Check sheet for the drawn part. Datum: minimum x, y, z corner. Units: mm. Coordinates: 2 decimals unless noted, no trailing zeros. Loops run counter-clockwise (first coordinate to the right, second up) from the corner with the lowest first, then second, coordinate; pieces in that order, holes last. Notation, with made-up numbers: (38.25, 60.25) - (64.25, 60.25) arc R9 cw to (64.25, 74.25) - close; hole circle Ø5 at (-19, 83.5). An arc over 180 degrees is marked (long way). Answer as CSV lines item,"result". Start each with the question number.
1. Gauge pin test, flat end, axial feed: P1, Ø1.8, axis at x = 2.5, y = 2.5, coming from the +Z side. Record the tip position at first contact, or that the pin passes through.
2. Cross-section at A-A (x = 2.5). Enter the section's corners in (y, z), plus the area to 3 significant figures.
3. Cross-section at B-B (z = 0.6). Enter the section's corners in (x, y), plus the area to 3 significant figures.
4. Cross-section at C-C (x = 3.75). Enter the section's corners in (y, z), plus the area to 3 significant figures.
5. Material ranges on line 1 (Y direction, x = 2.5, z = 1.4); line 2 (Y direction, x = 1.35, z = 1.85); line 3 (X direction, y = 3.5, z = 0.65), recorded low to high. Write a range as [from, to].
6. Release check for a two-part mould opening along Y. For the marked faces 1, 2 and 3 record: pulls with the +Y half, pulls with the -Y half, needs draft (parallel to the pull), parting line crosses it, or undercut.
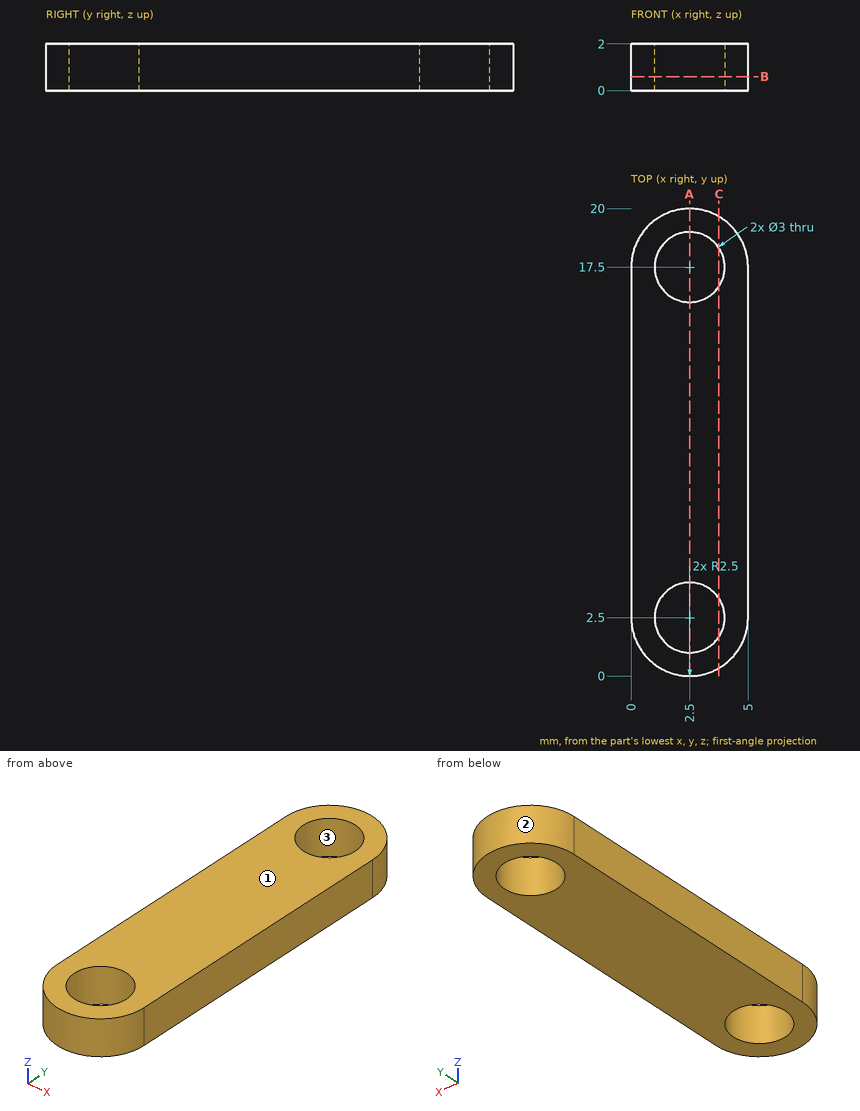
Values follow:
1,P1,"passes through"
2,outline,"(0, 0) - (1, 0) - (1, 2) - (0, 2) - close; (4, 0) - (16, 0) - (16, 2) - (4, 2) - close; (19, 0) - (20, 0) - (20, 2) - (19, 2) - close"
2,area,"28.0 mm²"
3,outline,"(0, 2.5) arc R2.5 ccw to (5, 2.5) - (5, 17.5) arc R2.5 ccw to (0, 17.5) - close; hole circle Ø3 at (2.5, 2.5); hole circle Ø3 at (2.5, 17.5)"
3,area,"80.5 mm²"
4,outline,"(0.33, 0) - (1.67, 0) - (1.67, 2) - (0.33, 2) - close; (3.33, 0) - (16.67, 0) - (16.67, 2) - (3.33, 2) - close; (18.33, 0) - (19.67, 0) - (19.67, 2) - (18.33, 2) - close"
4,area,"32.0 mm²"
5,line 1,"y = [0, 1], [4, 16], [19, 20]"
5,line 2,"y = [0.28, 1.54], [3.46, 16.54], [18.46, 19.72]"
5,line 3,"x = [0, 1.38], [3.62, 5]"
6,face 1,"needs draft"
6,face 2,"pulls with the +Y half"
6,face 3,"undercut"
